Here's how the part is built. I have some questions about the finished solid (model axes, mm). Face numbers are marked on the shaded views. A direction names the side the tool comes from. Give positions to 0.01 mm unless a question says otherwise; leave off trailing zeros. Loops run counter-clockwise (first coordinate to the right, second up) from the corner with the lowest first, then second, coordinate; pieces in that order, holes last. Notation, with made-up numbers: M 36,46 L 51,46 A27 cw 51,67 Z; hole C -31,32.5 d6. An arc over 180 degrees is marked long. Answer as CSV lines item,"result". Start each with the question number.
Item 1: Will these pins go through, and if not, where does the flat tip stop? P1, Ø3, axis at y = 2.5, z = 7, coming from the -X side; P2, Ø2, axis at x = -4, z = 5, coming from the -Y side; P3, Ø1, axis at y = 3, z = 7, coming from the -X side; P4, Ø2.5, axis at x = -2.5, y = -3.5, coming from the +Z side.
Item 2: I want a section at C-C on z = 4. List the corners of the cut face in (x, y) for me, plus the area to 3 significant figures.
Item 3: For the marked faces 1, 2 and 3, which set-ups out of +Z, -Z, +X, -X, +Y, -Y let a thin tool reach every point of the face, with its end or its side?
Item 4: I want a section at A-A on z = 5.75. List the corners of the cut face in (x, y) for me (3 decimals).
Item 5: If I drill on line 1 along Y through (x, z) = (0, 2.25); line 2 along Z through (x, y) = (2.5, 3), over which ranges is the centre line in solid material (lowest first)? Write a range as from..to.
Item 6: I want a section at B-B on y = 0. List the corners of the cut face in (x, z) for me.
Item 7: If we mould it in two halves opening along Y, with no side actions, what happens to the marked faces 4, 5 and 6? For each: released by +Y, released by -Y, zero draft, split by the parting line, or undercut.
Item 8: I want a section at D-D on y = 2. List the corners of the cut face in (x, z) for me, plus the area to 3 significant figures.
from build123d import *

# Parameters (mm, degrees)
PAD002_DEPTH = 10
PAD001_DEPTH = 10
SKETCH_R     = 5
SKETCH_R_2   = 3.2
PAD_DEPTH    = 12
FILLET_R     = 1


with BuildPart() as pad002:
    # Sketch002 → Pad002 (new body)
    with BuildSketch(Plane.XZ):
        Polygon((-5, 8), (0.75, 8), (0.75, 5), (3, 5), (3, 8), (5, 8), (5, 12), (-5, 12), align=None)
    extrude(amount=-PAD002_DEPTH)


with BuildPart() as pad001:
    # Sketch001 → Pad001 (new body)
    with BuildSketch(Plane.XZ):
        Polygon((5, 8), (5, 12), (-5, 12), (-5, 8), (-3, 8), (-3, 5), (-0.875, 5), (-0.875, 8), align=None)
    extrude(amount=PAD001_DEPTH)


with BuildPart() as fillet_body:
    # Sketch → Pad (new body)
    with BuildSketch(Plane.XY):
        Circle(SKETCH_R)
        Circle(SKETCH_R_2, mode=Mode.SUBTRACT)
    extrude(amount=PAD_DEPTH)

    # Cut: cut Pad001
    add(pad001.part, mode=Mode.SUBTRACT)

    # Cut001: cut Pad002
    add(pad002.part, mode=Mode.SUBTRACT)

    # Fillet
    fillet_edges = [fillet_body.edges().sort_by_distance(p)[0] for p in [
        (-0.875, -4.000445, 8),
        (0.75, 4.027149, 8),
    ]]
    fillet(fillet_edges, radius=FILLET_R)


solid = fillet_body.part
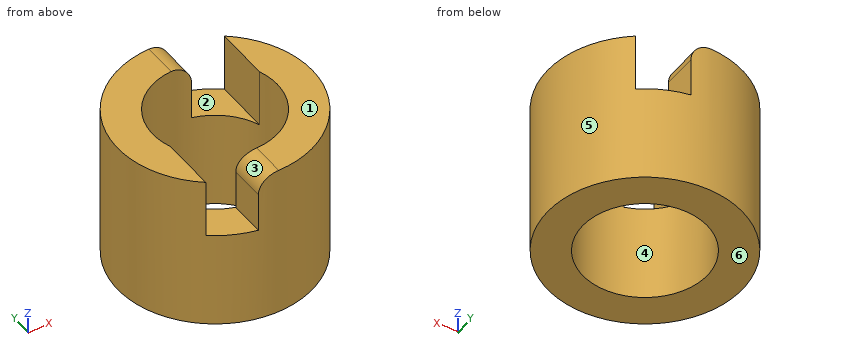
Result:
1,P1,"x = -4.9"
1,P2,"y = -4"
1,P3,"x = -4.33"
1,P4,"z = 8"
2,outline,"C 0,0 d10; hole C 0,0 d6.4"
2,area,"46.4 mm^2"
3,face 1,"+Z, +X, -X, +Y, -Y"
3,face 2,"+Z, +Y"
3,face 3,"+Z, -Y"
4,outline,"M -3,-4 L -3,-1.114 A3.2 cw 0.75,3.111 L 0.75,4.943 A5 ccw Z; M -0.875,-4.923 A5 ccw 3,4 L 3,1.114 A3.2 cw -0.875,-3.078 Z"
5,line 1,"-5..-3.2, 3.2..5"
5,line 2,"0..5"
6,outline,"M -5,0 L -3.2,0 L -3.2,8 L -5,8 Z; M 3.2,0 L 5,0 L 5,8 L 3.2,8 Z"
7,face 4,"undercut"
7,face 5,"split by the parting line"
7,face 6,"zero draft"
8,outline,"M -4.58,0 L -2.5,0 L -2.5,8 L -4.58,8 Z; M 2.5,0 L 4.58,0 L 4.58,8 L 3,8 L 3,5 L 2.5,5 Z"
8,area,"31.8 mm^2"
